from build123d import *

# Parameters (mm, degrees)
CROQUIS1_R              = 31.75
CROQUIS1_R_2            = 6.35
SALIENTE_EXTRUIR1_DEPTH = 19.05


with BuildPart() as part:
    # Croquis1 → Saliente-Extruir1 (new body)
    with BuildSketch(Plane.XY):
        Circle(CROQUIS1_R)
        Circle(CROQUIS1_R_2, mode=Mode.SUBTRACT)
    extrude(amount=SALIENTE_EXTRUIR1_DEPTH)

    # Croquis2 → Cortar-Revolución2 (revolve, cut)
    with BuildSketch(Plane(origin=(0, 0, 0), x_dir=(0, 0, -1), z_dir=(1, 0, 0))):
        Polygon((-3.042533403, 29.934999), (-16.007466597, 29.934999), (-17.05, 31.740719823), (-17.05, 32.934999), (-2, 32.934999), (-2, 31.740719823), align=None)
    revolve(axis=Axis((0, 0, 0), (0, 0, 1)), mode=Mode.SUBTRACT)


solid = part.part
The listing builds one solid part. Answer for the finished solid, in the listing's coordinates (mm). Round coordinates to 2 decimals unless told otherwise and drop trailing zeros. Order: outer loops, then holes, each group sorted by start corner. A loop starts at its lowest first (then second) coordinate and runs counter-clockwise, first axis right, second up. Notation, with made-up numbers: M -28.75,-20 L -14.75,-20 A17 ccw -14.75,1 Z; hole C 66,-31 d11. An arc over 180 degrees is marked long. Answer in a Markdown table with one row per item. Add a question column.
1) Consider line 1 along Y through (x, z) = (0, 14.5) (3 decimals); line 2 along Y through (x, z) = (2, 5); line 3 along Y through (x, z) = (16, 1.25). Determine where each line is inside the solid, lowest interval first. Write a range as from..to.
2) The part is cut by section A-A on y = 0. Determine the outline of the cut face in (x, z) (3 decimals), plus the area to 3 significant figures.
3) The part is cut by section C-C on z = 4.25. Determine the outline of the cut face in (x, y) (3 decimals).
4) Determine the mould class of faces 1 (the face through (-1.38, -6.2, 9.39)), 2 (the face through (18.21, -23.76, 9.62)), 3 (the face through (7, 0, 0)) for opening direction Z: pulls with the +Z half, pulls with the -Z half, needs draft (parallel to the pull), parting line crosses it, or undercut.
5) Flat-ended cylindrical pins translate along their axes: pin 1 Ø6 at (x, z) = (-14.5, 15.5) entering from -Y; pin 2 Ø4 at (x, z) = (19, 4) entering from +Y; pin 3 Ø10 at (y, z) = (-20.5, 10) entering from +X. Find the tip coordinate at first contact, or state that the pin passes through.
Findings below:
| question | item | result |
|---|---|---|
| 1 | line 1 | y = -29.935..-6.35, 6.35..29.935 |
| 1 | line 2 | y = -29.87..-6.03, 6.03..29.87 |
| 1 | line 3 | y = -27.42..27.42 |
| 2 | outline | M -31.75,0 L -6.35,0 L -6.35,19.05 L -31.75,19.05 L -31.75,17.05 L -31.741,17.05 L -29.935,16.007 L -29.935,3.043 L -31.741,2 L -31.75,2 Z; M 6.35,0 L 31.75,0 L 31.75,2 L 31.741,2 L 29.935,3.043 L 29.935,16.007 L 31.741,17.05 L 31.75,17.05 L 31.75,19.05 L 6.35,19.05 Z |
| 2 | area | 917 mm² |
| 3 | outline | C 0,0 d59.87; hole C 0,0 d12.7 |
| 4 | face 1 | needs draft |
| 4 | face 2 | undercut |
| 4 | face 3 | pulls with the -Z half |
| 5 | pin 1 | stops at y = -29.42 |
| 5 | pin 2 | stops at y = 25.67 |
| 5 | pin 3 | stops at x = 25.61 |
